Source: three-view drawing plus pictorial views. Frame: mm from the lowest corner of the part. A direction names the side the tool comes from. Give positions to 0.01 mm unless a question says otherwise; leave off trailing zeros. Loops run counter-clockwise (first coordinate to the right, second up) from the corner with the lowest first, then second, coordinate; pieces in that order, holes last. Notation, with made-up numbers: (-8, 66.5) - (38, 66.5) arc R18 cw to (38, 74.5) - close; hole circle Ø6 at (68, -7.5). An arc over 180 degrees is marked (long way). Answer in a Markdown table with one row per item.
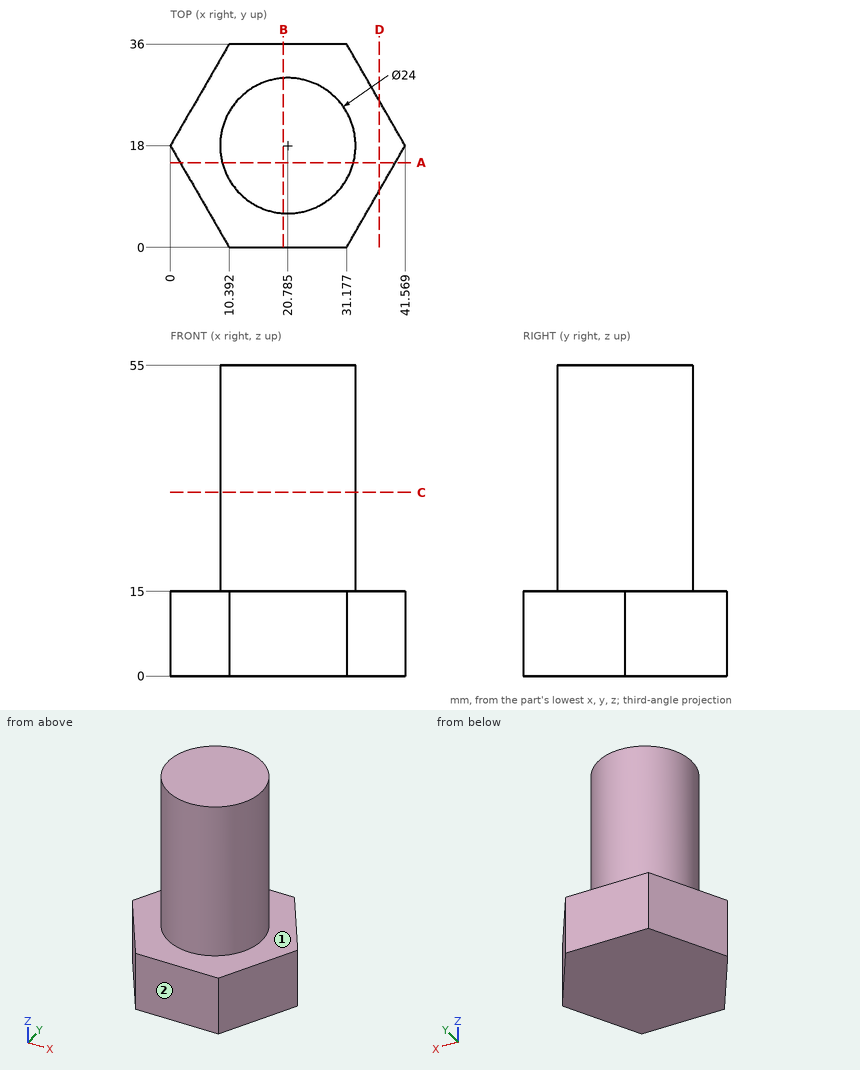
Q1. Cut plane A-A (y = 15). Output: boundary loops of the cut face in (x, z) (1 decimal).
Check values:
| item | result |
|---|---|
| outline | (1.7, 0) - (39.8, 0) - (39.8, 15) - (32.4, 15) - (32.4, 55) - (9.2, 55) - (9.2, 15) - (1.7, 15) - close |
Q2. Material intervals for line 1 along Z through (x, y) = (18, 33.5); line 2 along Y through (x, z) = (23.5, 35); line 3 along Y through (x, z) = (13, 26), sorted ascending.
Check values:
| item | result |
|---|---|
| line 1 | 0 to 15 |
| line 2 | 6.31 to 29.69 |
| line 3 | 8.87 to 27.13 |
Q3. First-contact query: pin 1 (3 mm diameter, centred on x = 12, z = 45, fed in from +Y) (1 decimal); pin 2 (1 mm diameter, centred on x = 34, y = 19, fed in from +Z); pin 3 (3 mm diameter, centred on y = 28.5, z = 36.5, fed in from -X). Flat tips, straight axial feed; report the tip coordinate or a pass-through.
Check values:
| item | result |
|---|---|
| pin 1 | y = 27.5 |
| pin 2 | z = 15 |
| pin 3 | x = 12.85 |
Q4. Cut plane C-C (z = 32.5). Output: boundary loops of the cut face in (x, y) (1 decimal).
Check values:
| item | result |
|---|---|
| outline | circle Ø24 at (20.8, 18) |
Q5. Cut plane B-B (x = 20). Output: boundary loops of the cut face in (y, z) (1 decimal), and give its area (3 significant figures).
Check values:
| item | result |
|---|---|
| outline | (0, 0) - (36, 0) - (36, 15) - (30, 15) - (30, 55) - (6, 55) - (6, 15) - (0, 15) - close |
| area | 1,500 mm² |
Q6. Cut plane D-D (x = 37). Output: boundary loops of the cut face in (y, z), and give its area (3 significant figures).
Check values:
| item | result |
|---|---|
| outline | (10.09, 0) - (25.91, 0) - (25.91, 15) - (10.09, 15) - close |
| area | 237 mm² |
Q7. Reachability of the marked faces 1 and 2 from +Z, -Z, +X, -X, +Y, -Y: full face, straight path, thin tool, end or side. Return the list, or none.
Check values:
| item | result |
|---|---|
| face 1 | +Z |
| face 2 | +Z, -Z, +X, -X, -Y |
